Design review of the part built by this model. Coordinates are the model's own, in mm. A direction names the side the tool comes from. Coordinates: 2 decimals unless noted, no trailing zeros. Write each loop counter-clockwise with the first axis right and the second up, starting at its lowest first coordinate (ties: lowest second). Pieces come first, ordered by that corner, then holes. Notation, with made-up numbers: (56.25, 68.25) - (79.25, 68.25) arc R17 ccw to (79.25, 97.25) - close; hole circle Ø4 at (-2.5, 64). An arc over 180 degrees is marked (long way). Use a Markdown table: item, result.
from build123d import *

# Parameters (mm, degrees)
F0_R     = 63.4990501998
F1_DEPTH = 127
F1_TAPER = -20
F2_R     = 25.4
F3_SIZE  = 63.5
F5_T     = -12.7


# Not quite as in the source:
# - a feature of the source that left no trace in its solid (it failed there, or was rolled back) is left out


with BuildPart() as f1:
    # F0 (on Front) → F1 (new body, symmetric)
    with BuildSketch(Plane.XZ):
        Circle(F0_R)
    extrude(amount=F1_DEPTH, both=True, taper=F1_TAPER)

    # F2
    f2_edges = [f1.edges().sort_by_distance(p)[0] for p in [
        (-63.49905, 0, 0),
        (-109.72327, -127, 0),
    ]]
    fillet(f2_edges, radius=F2_R)

    # F3
    f3_edges = [f1.edges().sort_by_distance(p)[0] for p in [
        (-109.72327, 127, 0),
    ]]
    chamfer(f3_edges, length=F3_SIZE)

    # F5
    f5_openings = [f1.faces().sort_by_distance(p)[0] for p in [
        (0, 127, 0),
    ]]
    offset(amount=F5_T, openings=f5_openings)


solid = f1.part
(1) Take a section at A-A on y = -54. Write out the cut boundary in (x, z).
Determined:
| item | result |
|---|---|
| outline | circle Ø166.31 at (0, 0); hole circle Ø139.28 at (0, 0) |
(2) For L1, parallel to Y at x = -54.5, z = 54; L2, parallel to Y at x = 58, z = -36; L3, parallel to Y at x = -39, z = 74, list the stretches that pass through material, from the lowest coordinate up. Write a range as from..to.
Determined:
| item | result |
|---|---|
| L1 | -126.79..-113.87, -73.46..-36.33, 36.33..83.44 |
| L2 | -127..-114.3, -50.22..-13.09, 13.09..50.22, 73.38..95.52 |
| L3 | -124.86..-109.17, -92.49..-55.36, 55.36..73.55 |
(3) Take a section at B-B on z = -60. State how many separate pieces and enclosed holes the cut face has, and give its area (3 significant figures).
Determined:
| item | result |
|---|---|
| separate pieces | 1 |
| enclosed holes | 2 |
| area | 13,400 mm2 |
(4) Take a section at C-C on y = 86. Write out the cut boundary in (x, z), and give its area (3 significant figures).
Determined:
| item | result |
|---|---|
| outline | circle Ø149.86 at (0, 0); hole circle Ø118.86 at (0, 0) |
| area | 6,540 mm2 |
(5) For pin 1 (12 mm diameter, centred on y = 91.5, z = -30.5, fed in from -X); pin 2 (3 mm diameter, centred on x = 31, z = -41.5, fed in from +Y); pin 3 (8 mm diameter, centred on y = 69.5, z = -12, fed in from +X), all flat-tipped, find the tip position at first contact; note any pin that passes through.
Determined:
| item | result |
|---|---|
| pin 1 | x = -69.48 |
| pin 2 | y = 121.18 |
| pin 3 | x = 87.58 |
(6) Draft analysis for pull direction Y (two halves, no side actions). For faces 3 (the flat face through (-1, -127, 1)), 4 (the conical face through (60.53, -37.02, 19.06)), 5 (the conical face through (44.573, 124.103, -18.481)), state which applies: +Y half, -Y half, draft (parallel to the pull), parting line (faces both ways), or undercut.
Determined:
| item | result |
|---|---|
| face 3 | -Y half |
| face 4 | undercut |
| face 5 | +Y half |
(7) Machinability: for faces 1 (the conical face through (51.656, 16.311, -21.418)), 2 (the flat face through (10, 127, -30)), which of the approach directions +Z, -Z, +X, -X, +Y, -Y give a long, thin tool a straight path to every point of the face, cutting with its end or side? Answer none if there is none.
Determined:
| item | result |
|---|---|
| face 1 | none |
| face 2 | +Z, -Z, +X, -X, +Y |
